```python
from build123d import *

# Parameters (mm, degrees)
BASE_EXTRUDE_DEPTH = 12.7
FILLET1_R          = 0.635


with BuildPart() as part:
    # Sketch1 → Base-Extrude (new, symmetric)
    with BuildSketch(Plane.XY):
        with BuildLine():
            Line((-6.35, 15.875), (-15.875, 15.875))
            Line((-15.875, 15.875), (-15.875, -15.875))
            Line((-15.875, -15.875), (-6.35, -15.875))
            Line((-6.35, -15.875), (-6.35, -14.605))
            Line((-6.35, -14.605), (-7.083234843, -13.335))
            Line((-7.083234843, -13.335), (-7.816469684, -14.605))
            Line((-7.816469684, -14.605), (-13.97, -14.605))
            ThreePointArc((-13.97, -14.605), (-14.419012806, -14.419012806), (-14.605, -13.97))
            Line((-14.605, -13.97), (-14.605, -8.5725))
            Line((-14.605, -8.5725), (-13.97, -8.5725))
            Line((-13.97, -8.5725), (-13.97, -7.3025))
            Line((-13.97, -7.3025), (-14.605, -7.3025))
            Line((-14.605, -7.3025), (-14.605, -1.27))
            ThreePointArc((-14.605, -1.27), (-14.419012806, -0.820987194), (-13.97, -0.635))
            Line((-13.97, -0.635), (13.97, -0.635))
            ThreePointArc((13.97, -0.635), (14.419012806, -0.820987194), (14.605, -1.27))
            Line((14.605, -1.27), (14.605, -7.3025))
            Line((14.605, -7.3025), (13.97, -7.3025))
            Line((13.97, -7.3025), (13.97, -8.5725))
            Line((13.97, -8.5725), (14.605, -8.5725))
            Line((14.605, -8.5725), (14.605, -13.97))
            ThreePointArc((14.605, -13.97), (14.419012806, -14.419012806), (13.97, -14.605))
            Line((13.97, -14.605), (7.816469684, -14.605))
            Line((7.816469684, -14.605), (7.083234843, -13.335))
            Line((7.083234843, -13.335), (6.35, -14.605))
            Line((6.35, -14.605), (6.35, -15.875))
            Line((6.35, -15.875), (15.875, -15.875))
            Line((15.875, -15.875), (15.875, 15.875))
            Line((15.875, 15.875), (6.35, 15.875))
            Line((6.35, 15.875), (6.35, 14.605))
            Line((6.35, 14.605), (7.083234843, 13.335))
            Line((7.083234843, 13.335), (7.816469684, 14.605))
            Line((7.816469684, 14.605), (13.97, 14.605))
            ThreePointArc((13.97, 14.605), (14.419012806, 14.419012806), (14.605, 13.97))
            Line((14.605, 13.97), (14.605, 8.5725))
            Line((14.605, 8.5725), (13.97, 8.5725))
            Line((13.97, 8.5725), (13.97, 7.3025))
            Line((13.97, 7.3025), (14.605, 7.3025))
            Line((14.605, 7.3025), (14.605, 1.27))
            ThreePointArc((14.605, 1.27), (14.419012806, 0.820987194), (13.97, 0.635))
            Line((13.97, 0.635), (-13.97, 0.635))
            ThreePointArc((-13.97, 0.635), (-14.419012806, 0.820987194), (-14.605, 1.27))
            Line((-14.605, 1.27), (-14.605, 7.3025))
            Line((-14.605, 7.3025), (-13.97, 7.3025))
            Line((-13.97, 7.3025), (-13.97, 8.5725))
            Line((-13.97, 8.5725), (-14.605, 8.5725))
            Line((-14.605, 8.5725), (-14.605, 13.97))
            ThreePointArc((-14.605, 13.97), (-14.419012806, 14.419012806), (-13.97, 14.605))
            Line((-13.97, 14.605), (-7.816469684, 14.605))
            Line((-7.816469684, 14.605), (-7.083234843, 13.335))
            Line((-7.083234843, 13.335), (-6.35, 14.605))
            Line((-6.35, 14.605), (-6.35, 15.875))
        make_face()
    extrude(amount=BASE_EXTRUDE_DEPTH, both=True)

    # Fillet1
    fillet1_edges = [part.edges().sort_by_distance(p)[0] for p in [
        (14.605, 8.5725, 0),
        (14.605, -7.3025, 0),
        (-14.605, 8.5725, 0),
        (-14.605, -7.3025, 0),
        (-14.605, 7.3025, 0),
        (-14.605, -8.5725, 0),
        (14.605, 7.3025, 0),
        (14.605, -8.5725, 0),
    ]]
    fillet(fillet1_edges, radius=FILLET1_R - 0.0001)  # a hair under: the kernel refuses the full size


solid = part.part
```
Here's how the part is built. I have some questions about the finished solid (model axes, mm). A direction names the side the tool comes from. Give positions to 0.01 mm unless a question says otherwise; leave off trailing zeros. Loops run counter-clockwise (first coordinate to the right, second up) from the corner with the lowest first, then second, coordinate; pieces in that order, holes last. Notation, with made-up numbers: M -22.75,-0.5 L 32.25,-0.5 A17 cw 32.25,6.5 Z; hole C 82,39 d9. An arc over 180 degrees is marked long. Use one line per item in the form item = value. Start each with the question number.
Q1. If we section it at A-A (y = -12): Write out the boundary of the cut face in (x, z) (3 decimals), then the cut area to 3 significant figures.
Q2. Will these pins go through, and if not, where does the flat tip stop? pin 1 Ø6 at (x, z) = (-2.5, -7) entering from +Y (3 decimals); pin 2 Ø2 at (x, z) = (-5, 7) entering from -Y (3 decimals).
Q3. If we section it at B-B (x = 9): Write out the boundary of the cut face in (y, z) (3 decimals).
Q4. Thinking about a two-plate mould opening in Z: for faces 1 (the flat face through (0, 0, 12.7)), 2 (the flat face through (0, 0, -12.7)), 3 (the flat face through (14.605, 12, 0)), which applies, +Z half, -Z half, draft (parallel to the pull), parting line (faces both ways), or undercut?
Q5. Which directions (+Z, -Z, +X, -X, +Y, -Y) give clear straight access to the entire face, cutting with the end or side of a thin tool? Please do faces 4 (the flat face through (0, 0.635, 0)), 5 (the flat face through (6.35, 15, 0)), 6 (the flat face through (-11, -15.875, 0)).
Q6. I need wall thicknesses on line 1 along Y through (x, z) = (-9, -3.75) (3 decimals); line 2 along X through (y, z) = (-4, -8.25) (3 decimals); line 3 along X through (y, z) = (14, 9.75) (3 decimals). Which ranges of each line are inside material? Lowest first, please.
Q7. If we section it at C-C (x = -0.5): Write out the boundary of the cut face in (y, z) (3 decimals).
Taken from the geometry:
q1.outline = M -15.875,-12.7 L -14.605,-12.7 L -14.605,12.7 L -15.875,12.7 Z; M 14.605,-12.7 L 15.875,-12.7 L 15.875,12.7 L 14.605,12.7 Z
q1.area = 64.5 mm^2
q2.pin_1 = 0.635
q2.pin_2 = -0.635
q3.outline = M -15.875,-12.7 L -14.605,-12.7 L -14.605,12.7 L -15.875,12.7 Z; M -0.635,-12.7 L 0.635,-12.7 L 0.635,12.7 L -0.635,12.7 Z; M 14.605,-12.7 L 15.875,-12.7 L 15.875,12.7 L 14.605,12.7 Z
q4.face_1 = +Z half
q4.face_2 = -Z half
q4.face_3 = draft
q5.face_4 = +Z, -Z
q5.face_5 = +Z, -Z, +Y
q5.face_6 = +Z, -Z, +X, -X, -Y
q6.line_1 = -15.875 to -14.605, -0.635 to 0.635, 14.605 to 15.875
q6.line_2 = -15.875 to -14.605, 14.605 to 15.875
q6.line_3 = -15.875 to -14.604, -7.467 to -6.699, 6.699 to 7.467, 14.604 to 15.875
q7.outline = M -0.635,-12.7 L 0.635,-12.7 L 0.635,12.7 L -0.635,12.7 Z
